```python
from build123d import *

# Parameters (mm, degrees)
PAD005_DEPTH           = 0.1
SKETCH009_R            = 0.4
PAD006_DEPTH           = 15
LINEARPATTERN003_COUNT = 4
LINEARPATTERN003_PITCH = 2.54


with BuildPart() as part:
    # Sketch010 → Pad005 (new body)
    with BuildSketch(Plane.XY):
        with BuildLine():
            ThreePointArc((-17.25, 3.81), (-17.65, 4.21), (-18.05, 3.81))
            Line((-18.05, 3.81), (-18.05, -3.81))
            ThreePointArc((-18.05, -3.81), (-17.65, -4.21), (-17.25, -3.81))
            Line((-17.25, 3.81), (-17.25, -3.81))
        make_face()
    extrude(amount=PAD005_DEPTH)

    # Sketch009 → Pad006 (join)
    with BuildSketch(Plane.XY):
        with Locations((-17.65, -3.81)):
            Circle(SKETCH009_R)
    pad006 = extrude(amount=-PAD006_DEPTH)

    # LinearPattern003: Pad006 ×4
    with Locations(*[(0, i * LINEARPATTERN003_PITCH, 0) for i in range(1, LINEARPATTERN003_COUNT)]):
        add(pad006)


solid = part.part
```
Can you work these out from the model? Positions are in its coordinate system, mm. Give positions to 0.01 mm unless a question says otherwise; leave off trailing zeros. Loops run counter-clockwise (first coordinate to the right, second up) from the corner with the lowest first, then second, coordinate; pieces in that order, holes last. Notation, with made-up numbers: M 56.5,67 L 103.5,67 A13 ccw 103.5,92 Z; hole C 57.5,28 d7. An arc over 180 degrees is marked long. Use one line per item in the form item = value. Start each with the question number.
(1) I want a section at A-A, the plane z = -8.25. Write out the boundary of the cut face in (x, y), and give its area (3 significant figures).
(2) Please list where these lines run through material, in increasing order: line 1 (Y direction, x = -17.6, z = -6.5); line 2 (Y direction, x = -17.8, z = -1); line 3 (X direction, y = 1, z = -5.5).
(3) I want a section at C-C, the plane y = -2.75. Write out the boundary of the cut face in (x, z), and give its area (3 significant figures).
(4) I want a section at B-B, the plane x = -17.65. Write out the boundary of the cut face in (y, z).
Worked out:
q1.outline = C -17.65,-3.81 d0.8; C -17.65,-1.27 d0.8; C -17.65,1.27 d0.8; C -17.65,3.81 d0.8
q1.area = 2.01 mm²
q2.line_1 = -4.21 to -3.41, -1.67 to -0.87, 0.87 to 1.67, 3.41 to 4.21
q2.line_2 = -4.18 to -3.44, -1.64 to -0.9, 0.9 to 1.64, 3.44 to 4.18
q2.line_3 = -17.95 to -17.35
q3.outline = M -18.05,0 L -17.25,0 L -17.25,0.1 L -18.05,0.1 Z
q3.area = 0.0800 mm²
q4.outline = M -4.21,-15 L -3.41,-15 L -3.41,0 L -1.67,0 L -1.67,-15 L -0.87,-15 L -0.87,0 L 0.87,0 L 0.87,-15 L 1.67,-15 L 1.67,0 L 3.41,0 L 3.41,-15 L 4.21,-15 L 4.21,0.1 L -4.21,0.1 Z
